from build123d import *

# Parameters (mm, degrees)
EXTRUDE_1_DEPTH     = 129
SKETCH_2_R          = 2.25
CUT_EXTRUDE_1_DEPTH = 6
CUT_EXTRUDE_START   = -6
SKETCH_3_R          = 2.25
CUT_EXTRUDE_2_DEPTH = 6


with BuildPart() as part:
    # Эскиз1 → Бобышка-Вытянуть1 (new body)
    with BuildSketch(Plane.XY):
        with BuildLine():
            Line((3.75277675, 0.5), (2.309401077, 3))
            ThreePointArc((2.309401077, 3), (1.943375673, 3.366025404), (1.443375673, 3.5))
            Line((1.443375673, 3.5), (-1.443375673, 3.5))
            ThreePointArc((-1.443375673, 3.5), (-1.943375673, 3.366025404), (-2.309401077, 3))
            Line((-2.309401077, 3), (-3.75277675, 0.5))
            ThreePointArc((-3.75277675, 0.5), (-3.886751346, 0), (-3.75277675, -0.5))
            Line((-3.75277675, -0.5), (-2.309401077, -3))
            ThreePointArc((-2.309401077, -3), (-1.943375673, -3.366025404), (-1.443375673, -3.5))
            Line((-1.443375673, -3.5), (1.443375673, -3.5))
            ThreePointArc((1.443375673, -3.5), (1.943375673, -3.366025404), (2.309401077, -3))
            Line((2.309401077, -3), (3.75277675, -0.5))
            ThreePointArc((3.75277675, -0.5), (3.886751346, 0), (3.75277675, 0.5))
        make_face()
    extrude(amount=EXTRUDE_1_DEPTH)

    # Эскиз2 → Вырез-Вытянуть1 (cut)
    with BuildSketch(Plane.XY.offset(129)):
        Circle(SKETCH_2_R)
    extrude(amount=-CUT_EXTRUDE_1_DEPTH, mode=Mode.SUBTRACT)

    # Эскиз3 → Вырез-Вытянуть2 (cut)
    with BuildSketch(Plane(origin=(0, 0, 0), x_dir=(-1, 0, 0), z_dir=(0, 0, -1)).offset(CUT_EXTRUDE_START)):
        with Locations(Location((0, 0, 0), (0, 0, 180))):
            Circle(SKETCH_3_R)
    extrude(amount=CUT_EXTRUDE_2_DEPTH, mode=Mode.SUBTRACT)


solid = part.part
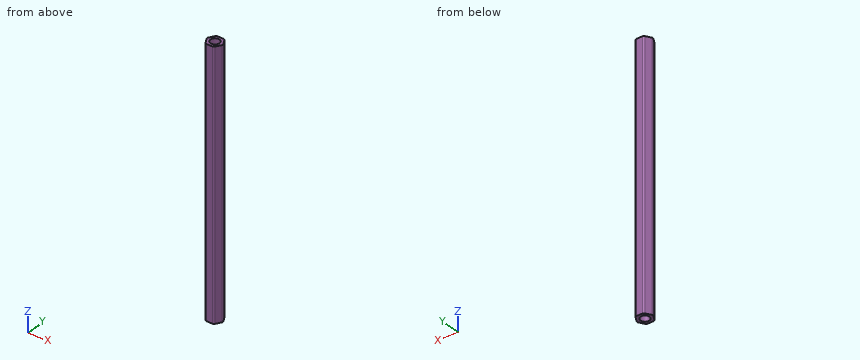
Source: CAD feature listing. Evaluate the final solid. Frame: model axes, mm. Round coordinates to 2 decimals unless told otherwise and drop trailing zeros. Loops run counter-clockwise (first coordinate to the right, second up) from the corner with the lowest first, then second, coordinate; pieces in that order, holes last. Notation, with made-up numbers: M 79.5,-26 L 85.5,-26 A19 cw 85.5,-3 Z; hole C 47,65.5 d2. An arc over 180 degrees is marked long. Return JSON: item names as keys, results as strings. Group by question number.
1. Pin query (flat end, axial travel): pin 1 (1 mm diameter, centred on y = -2.5, z = 31, fed in from +X); pin 2 (2.5 mm diameter, centred on x = 0, y = 0, fed in from +Z); pin 3 (1.3 mm diameter, centred on x = -1, y = 0, fed in from -Z). Return the tip coordinate at first contact, or that it passes through.
2. Section query B-B on z = 10.5. Output: boundary loops of the cut face in (x, y).
3. Material intervals for line 1 along Y through (x, z) = (0, 126.8); line 2 along Y through (x, z) = (-1.5, 81); line 3 along Z through (x, y) = (-2, 0.25), sorted ascending. Write a range as from..to.
4. Section query A-A on x = 0. Output: boundary loops of the cut face in (y, z), and give its area (3 significant figures).
Checks:
{
 "1": {"pin 1": "stops at x = 2.89", "pin 2": "stops at z = 123", "pin 3": "stops at z = 6"},
 "2": {"outline": "M -3.75,-0.5 L -2.31,-3 A1 ccw -1.44,-3.5 L 1.44,-3.5 A1 ccw 2.31,-3 L 3.75,-0.5 A1 ccw 3.75,0.5 L 2.31,3 A1 ccw 1.44,3.5 L -1.44,3.5 A1 ccw -2.31,3 L -3.75,0.5 A1 ccw Z"},
 "3": {"line 1": "y = -3.5..-2.25, 2.25..3.5", "line 2": "y = -3.5..3.5", "line 3": "z = 6..123"},
 "4": {"outline": "M -3.5,0 L -2.25,0 L -2.25,6 L 2.25,6 L 2.25,0 L 3.5,0 L 3.5,129 L 2.25,129 L 2.25,123 L -2.25,123 L -2.25,129 L -3.5,129 Z", "area": "849 mm²"}
}
